Model file for the job. Use its own axes, mm. Face numbers are marked on the shaded views. A direction names the side the tool comes from. Round coordinates to 2 decimals unless told otherwise and drop trailing zeros. Order: outer loops, then holes, each group sorted by start corner. A loop starts at its lowest first (then second) coordinate and runs counter-clockwise, first axis right, second up. Notation, with made-up numbers: (39, 15) - (92, 15) arc R9 cw to (92, 21) - close; hole circle Ø3 at (28, 46.25). An arc over 180 degrees is marked (long way). Answer as CSV lines item,"result". Start each with the question number.
1. 3-axis set-ups, long thin cutter, end or side, ignore diameter. For the marked faces 1 and 2: which of +Z, -Z, +X, -X, +Y, -Y reach the whole face in a straight line?
2. Pin check, flat tips, straight feed: pin 1 Ø1.5 at (x, z) = (-0.5, -13.5) entering from -Y; pin 2 Ø3 at (y, z) = (-2, -16) entering from +X; pin 3 Ø0.6 at (x, z) = (0, 1) entering from -Y. Stop position of each tip, or through.
3. Band-saw the part on B-B on z = -14.25. List the corners of the cut face in (x, y).
4. Band-saw the part on A-A on x = 0. List the corners of the cut face in (y, z), then the cut area to 3 significant figures.
5. Wall check: line 1 along Z through (x, y) = (0, 3); line 2 along Y through (x, z) = (0, -18); line 3 along Z through (x, y) = (0.5, 0.5). Give the ranges that are in metal, low to high. Write a range as [from, to].
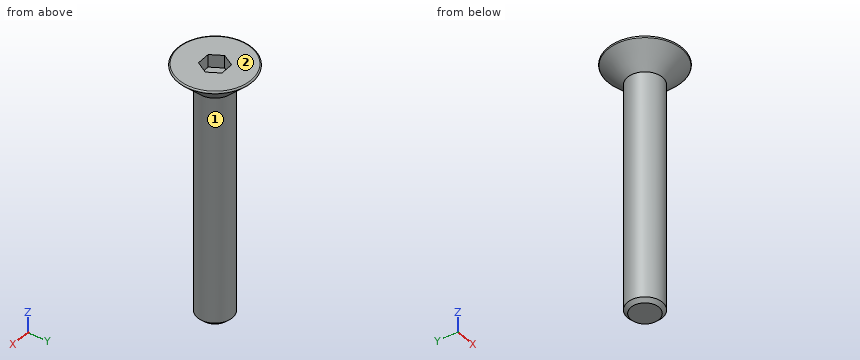
Autodesk Inventor part; units mm, degrees
ref_plane "YZ Plane" through (0, 0, 0) normal (1, 0, 0) x (0, 1, 0)
ref_plane "XZ Plane" through (0, 0, 0) normal (0, 1, 0) x (-1, 0, 0)
ref_plane "XY Plane" through (0, 0, 0) normal (0, 0, 1) x (1, 0, 0)
sketch "Sketch2" plane through (0, 0, 0) normal (0, 0, 1) x (1, 0, 0)
  circle A0 centre (0, 0) radius 1.5
  dimension "Diameter" = 3
extrude "Extrusion1" add sketch "Sketch2" against normal blind 20
sketch "Sketch3" plane through (0, 0, 0) normal (0, 0, 1) x (1, 0, 0)
  circle A0 centre (0, 0) radius 1.5
extrude "Extrusion2" add sketch "Sketch3" along normal blind 1.86 draft 45
sketch "Sketch4" plane through (0, 0, 1.86) normal (0, 0, 1) x (1, 0, 0)
  circle A0 centre (0, 0) radius 3.36
  line L0 (0.5774, 1) -> (1.1547, 0)
  line L1 (1.1547, 0) -> (0.5774, -1)
  line L2 (0.5774, -1) -> (-0.5774, -1)
  line L3 (-0.5774, -1) -> (-1.1547, 0)
  line L4 (-1.1547, 0) -> (-0.5774, 1)
  line L5 (-0.5774, 1) -> (0.5774, 1)
  line L6 (0, 0) -> (1.1547, 0) construction
  dimension "Hex_Width" = 2
extrude "Extrusion3" cut sketch "Sketch4" against normal blind 1.1 contours L0 L1 L2 L3 L4 L5
thread "Thread1"
chamfer "Chamfer1" distance 0.3 angle 45 1 edges at (-1.5, 0, -20)
fillet "Fillet1" radius 0.1 1 edges at (-3.36, 0, 1.86)
equation "\"Thread_Length\" = Length1"
properties part number "SCREW,FLAT-HD,P,10_9,M03X0_50X20MM" material "Steel, MS"
Reply:
1,face 1,"-Z"
1,face 2,"+Z, +X, -X, +Y, -Y"
2,pin 1,"stops at y = -1.5"
2,pin 2,"stops at x = 1.41"
2,pin 3,"stops at y = -2.8"
3,outline,"circle Ø3 at (0, 0)"
4,outline,"(-3.19, 1.69) - (-1.5, 0) - (-1.5, -19.7) - (-1.2, -20) - (1.2, -20) - (1.5, -19.7) - (1.5, 0) - (3.19, 1.69) arc R0.1 ccw to (3.12, 1.86) - (1, 1.86) - (1, 0.76) - (-1, 0.76) - (-1, 1.86) - (-3.12, 1.86) arc R0.1 ccw to start"
4,area,"66.7 mm2"
5,line 1,"z = [1.5, 1.86]"
5,line 2,"y = [-1.5, 1.5]"
5,line 3,"z = [-20, 0.76]"
